```python
from build123d import *

# Parameters (mm, degrees)
ESQUISSE1_R        = 6.5
ESQUISSE1_R_2      = 2.5
BOSS_EXTRU_1_DEPTH = 5
ESQUISSE2_R        = 7.5
ESQUISSE2_R_2      = 3
BOSS_EXTRU_2_DEPTH = 1
CHANFREIN1_SIZE    = 0.25


with BuildPart() as part:
    # Esquisse1 → Boss.-Extru.1 (new body)
    with BuildSketch(Plane.XY):
        Circle(ESQUISSE1_R)
        Circle(ESQUISSE1_R_2, mode=Mode.SUBTRACT)
    extrude(amount=BOSS_EXTRU_1_DEPTH)

    # Esquisse2 → Boss.-Extru.2 (add)
    with BuildSketch(Plane.XY.offset(5)):
        Circle(ESQUISSE2_R)
        Circle(ESQUISSE2_R_2, mode=Mode.SUBTRACT)
    extrude(amount=-BOSS_EXTRU_2_DEPTH)

    # Chanfrein1
    chanfrein1_edges = [part.edges().sort_by_distance(p)[0] for p in [
        (-7.5, 0, 5),
        (-6.5, 0, 0),
        (-2.5, 0, 5),
    ]]
    chamfer(chanfrein1_edges, length=CHANFREIN1_SIZE)


solid = part.part
```
Source: CAD feature listing. Evaluate the final solid. Frame: model axes, mm. A direction names the side the tool comes from. Coordinates: 2 decimals unless noted, no trailing zeros. Loops run counter-clockwise (first coordinate to the right, second up) from the corner with the lowest first, then second, coordinate; pieces in that order, holes last. Notation, with made-up numbers: M 64.25,-6 L 106.25,-6 A12 cw 106.25,6 Z; hole C 53,53.5 d2. An arc over 180 degrees is marked long. Put each result on its own line as item: value. Start each with the question number.
1) Cut plane C-C on z = 2.4. Return the cut outline in (x, y).
2) Pull-direction query (X, two-part tool) for faces 1 (the face through (-6, 3, 4)), 2 (the face through (-0.54, -2.44, 2.34)), 3 (the face through (-7.493, 0.33, 4.38)); classes: pulls with the +X half, pulls with the -X half, needs draft (parallel to the pull), parting line crosses it, or undercut.
3) Cut plane A-A on x = 0. Return the cut outline in (y, z), then the cut area to 3 significant figures.
4) Contact query for flat-ended pins moving along their axis: pin 1 Ø1.5 at (x, z) = (0.5, 2.5) entering from -Y; pin 2 Ø4 at (x, y) = (0, 0) entering from -Z. Output: stop coordinate, or through.
5) Reachability of faces 4 (the face through (-5.158, -3.955, 2.099)), 5 (the face through (3, 0, 5)) from +Z, -Z, +X, -X, +Y, -Y: full face, straight path, thin tool, end or side. Return the list, or none.
6) Ray query, L1, parallel to Y at x = 0, z = 3.6; L2, parallel to Y at x = -1.25, z = 3.1; L3, parallel to X at y = 2, z = 2.15. Return the intervals inside material, ascending. Write a range as from..to.
The answers:
1. outline: C 0,0 d13; hole C 0,0 d5
2. face 1: needs draft
2. face 2: undercut
2. face 3: parting line crosses it
3. outline: M -7.5,4 L -6.5,4 L -6.5,0.25 L -6.25,0 L -2.5,0 L -2.5,4.75 L -2.75,5 L -7.25,5 L -7.5,4.75 Z; M 2.5,0 L 6.25,0 L 6.5,0.25 L 6.5,4 L 7.5,4 L 7.5,4.75 L 7.25,5 L 2.75,5 L 2.5,4.75 Z
3. area: 41.8 mm²
4. pin 1: stops at y = -6.5
4. pin 2: passes through
5. face 4: -Z
5. face 5: +Z, +X, -X, +Y, -Y
6. L1: y = -6.5..-2.5, 2.5..6.5
6. L2: y = -6.38..-2.17, 2.17..6.38
6. L3: x = -6.18..-1.5, 1.5..6.18
